Geometry check sheet. Reference: the model listing, model coordinates, mm. A direction names the side the tool comes from. Coordinates: 2 decimals unless noted, no trailing zeros. Order: outer loops, then holes, each group sorted by start corner. A loop starts at its lowest first (then second) coordinate and runs counter-clockwise, first axis right, second up.
```python
from build123d import *

# Parameters (mm, degrees)
SKETCH2_R           = 8
SKETCH2_R_2         = 1.6
SKETCH2_R_3         = 1.5
BOSS_EXTRUDE1_DEPTH = 3


with BuildPart() as part:
    # Sketch2 → Boss-Extrude1 (new body)
    with BuildSketch(Plane.XY):
        with BuildLine():
            Line((118.698481804, 213.752755906), (168.691338583, 213.752755906))
            Line((168.691338583, 213.752755906), (178.691338583, 219.752755906))
            Line((178.691338583, 219.752755906), (258.691338583, 219.752755906))
            Line((258.691338583, 219.752755906), (268.691338583, 213.752755906))
            Line((268.691338583, 213.752755906), (338.214919991, 213.752755906))
            ThreePointArc((338.214919991, 213.752755906), (368.691338583, 289.752755906), (338.214919991, 365.752755906))
            Line((338.214919991, 365.752755906), (268.691338583, 365.752755906))
            Line((268.691338583, 365.752755906), (258.691338583, 359.752755906))
            Line((258.691338583, 359.752755906), (178.691338583, 359.752755906))
            Line((178.691338583, 359.752755906), (168.691338583, 365.752755906))
            Line((168.691338583, 365.752755906), (118.698481804, 365.752755906))
            ThreePointArc((118.698481804, 365.752755906), (111.678103304, 362.874152237), (108.699502265, 355.895613048))
            ThreePointArc((108.699502265, 355.895613048), (109.530508537, 343.195810526), (112.36497097, 330.788499042))
            ThreePointArc((112.36497097, 330.788499042), (123.691338583, 289.752755906), (112.36497097, 248.717012769))
            ThreePointArc((112.36497097, 248.717012769), (109.530508537, 236.309701285), (108.699502265, 223.609898763))
            ThreePointArc((108.699502265, 223.609898763), (111.678103304, 216.631359574), (118.698481804, 213.752755906))
        make_face()
        with Locations((198.291338583, 289.752755906)):
            Circle(SKETCH2_R, mode=Mode.SUBTRACT)
        with Locations((264.091338583, 289.752755906)):
            Circle(SKETCH2_R, mode=Mode.SUBTRACT)
        with Locations((264.091338583, 338.052755906)):
            Circle(SKETCH2_R_2, mode=Mode.SUBTRACT)
        with Locations((260.591338583, 318.752755906)):
            Circle(SKETCH2_R_2, mode=Mode.SUBTRACT)
        with Locations((245.391338583, 311.552755906)):
            Circle(SKETCH2_R_2, mode=Mode.SUBTRACT)
        with Locations((238.791338583, 344.752755906)):
            Circle(SKETCH2_R_2, mode=Mode.SUBTRACT)
        with Locations((239.591338583, 318.752755906)):
            Circle(SKETCH2_R_2, mode=Mode.SUBTRACT)
        with Locations((234.591338583, 312.752755906)):
            Circle(SKETCH2_R_2, mode=Mode.SUBTRACT)
        with Locations((227.791338583, 312.752755906)):
            Circle(SKETCH2_R_2, mode=Mode.SUBTRACT)
        with Locations((216.991338583, 311.552755906)):
            Circle(SKETCH2_R_2, mode=Mode.SUBTRACT)
        with Locations((222.791338583, 318.752755906)):
            Circle(SKETCH2_R_2, mode=Mode.SUBTRACT)
        with Locations((223.591338583, 344.752755906)):
            Circle(SKETCH2_R_2, mode=Mode.SUBTRACT)
        with Locations((201.791338583, 318.752755906)):
            Circle(SKETCH2_R_2, mode=Mode.SUBTRACT)
        with Locations((194.791338583, 318.752755906)):
            Circle(SKETCH2_R_2, mode=Mode.SUBTRACT)
        with Locations((199.100829472, 338.052755906)):
            Circle(SKETCH2_R_2, mode=Mode.SUBTRACT)
        with Locations((191.091338583, 320.252755906)):
            Circle(SKETCH2_R_2, mode=Mode.SUBTRACT)
        with Locations((191.091338583, 314.852755906)):
            Circle(SKETCH2_R_2, mode=Mode.SUBTRACT)
        with Locations((179.591338583, 311.552755906)):
            Circle(SKETCH2_R_2, mode=Mode.SUBTRACT)
        with Locations((173.791338583, 318.752755906)):
            Circle(SKETCH2_R_2, mode=Mode.SUBTRACT)
        with Locations((168.791338583, 312.752755906)):
            Circle(SKETCH2_R_2, mode=Mode.SUBTRACT)
        with Locations((163.691338583, 314.752755906)):
            Circle(SKETCH2_R_3, mode=Mode.SUBTRACT)
        with Locations((163.691338583, 326.752755906)):
            Circle(SKETCH2_R_3, mode=Mode.SUBTRACT)
        with Locations((163.691338583, 338.752755906)):
            Circle(SKETCH2_R_3, mode=Mode.SUBTRACT)
        with Locations((172.991338583, 344.752755906)):
            Circle(SKETCH2_R_2, mode=Mode.SUBTRACT)
        with Locations((163.691338583, 350.752755906)):
            Circle(SKETCH2_R_3, mode=Mode.SUBTRACT)
        with Locations((133.691338583, 350.752755906)):
            Circle(SKETCH2_R_3, mode=Mode.SUBTRACT)
        with Locations((120.691338583, 358.752755906)):
            Circle(SKETCH2_R_3, mode=Mode.SUBTRACT)
        with Locations((117.691338583, 341.752755906)):
            Circle(SKETCH2_R_3, mode=Mode.SUBTRACT)
        with Locations((133.691338583, 338.752755906)):
            Circle(SKETCH2_R_3, mode=Mode.SUBTRACT)
        with Locations((133.691338583, 326.752755906)):
            Circle(SKETCH2_R_3, mode=Mode.SUBTRACT)
        with Locations((133.691338583, 314.752755906)):
            Circle(SKETCH2_R_3, mode=Mode.SUBTRACT)
        with Locations((198.291338583, 241.452755906)):
            Circle(SKETCH2_R_2, mode=Mode.SUBTRACT)
        with Locations((201.791338583, 260.752755906)):
            Circle(SKETCH2_R_2, mode=Mode.SUBTRACT)
        with Locations((216.991338583, 267.952755906)):
            Circle(SKETCH2_R_2, mode=Mode.SUBTRACT)
        with Locations((227.791338583, 266.752755906)):
            Circle(SKETCH2_R_2, mode=Mode.SUBTRACT)
        with Locations((222.791338583, 260.752755906)):
            Circle(SKETCH2_R_2, mode=Mode.SUBTRACT)
        with Locations((223.591338583, 234.752755906)):
            Circle(SKETCH2_R_2, mode=Mode.SUBTRACT)
        with Locations((238.791338583, 234.752755906)):
            Circle(SKETCH2_R_2, mode=Mode.SUBTRACT)
        with Locations((234.591338583, 266.752755906)):
            Circle(SKETCH2_R_2, mode=Mode.SUBTRACT)
        with Locations((245.391338583, 267.952755906)):
            Circle(SKETCH2_R_2, mode=Mode.SUBTRACT)
        with Locations((239.591338583, 260.752755906)):
            Circle(SKETCH2_R_2, mode=Mode.SUBTRACT)
        with Locations((264.091338583, 241.452755906)):
            Circle(SKETCH2_R_2, mode=Mode.SUBTRACT)
        with Locations((260.591338583, 260.752755906)):
            Circle(SKETCH2_R_2, mode=Mode.SUBTRACT)
        with Locations((267.591338583, 260.752755906)):
            Circle(SKETCH2_R_2, mode=Mode.SUBTRACT)
        with Locations((271.291338583, 264.652755906)):
            Circle(SKETCH2_R_2, mode=Mode.SUBTRACT)
        with Locations((271.291338583, 259.252755906)):
            Circle(SKETCH2_R_2, mode=Mode.SUBTRACT)
        with Locations((289.391338583, 234.752755906)):
            Circle(SKETCH2_R_2, mode=Mode.SUBTRACT)
        with Locations((298.691338583, 228.752755906)):
            Circle(SKETCH2_R_3, mode=Mode.SUBTRACT)
        with Locations((298.691338583, 240.752755906)):
            Circle(SKETCH2_R_3, mode=Mode.SUBTRACT)
        with Locations((288.591338583, 260.752755906)):
            Circle(SKETCH2_R_2, mode=Mode.SUBTRACT)
        with Locations((282.791338583, 267.952755906)):
            Circle(SKETCH2_R_2, mode=Mode.SUBTRACT)
        with Locations((293.591338583, 266.752755906)):
            Circle(SKETCH2_R_2, mode=Mode.SUBTRACT)
        with Locations((298.691338583, 264.752755906)):
            Circle(SKETCH2_R_3, mode=Mode.SUBTRACT)
        with Locations((298.691338583, 252.752755906)):
            Circle(SKETCH2_R_3, mode=Mode.SUBTRACT)
        with Locations((328.691338583, 228.752755906)):
            Circle(SKETCH2_R_3, mode=Mode.SUBTRACT)
        with Locations((328.691338583, 240.752755906)):
            Circle(SKETCH2_R_3, mode=Mode.SUBTRACT)
        with Locations((328.691338583, 252.752755906)):
            Circle(SKETCH2_R_3, mode=Mode.SUBTRACT)
        with Locations((328.691338583, 264.752755906)):
            Circle(SKETCH2_R_3, mode=Mode.SUBTRACT)
        with Locations((350.691338583, 244.752755906)):
            Circle(SKETCH2_R_3, mode=Mode.SUBTRACT)
        with Locations((350.691338583, 334.752755906)):
            Circle(SKETCH2_R_3, mode=Mode.SUBTRACT)
        with Locations((328.691338583, 350.752755906)):
            Circle(SKETCH2_R_3, mode=Mode.SUBTRACT)
        with Locations((328.691338583, 338.752755906)):
            Circle(SKETCH2_R_3, mode=Mode.SUBTRACT)
        with Locations((328.691338583, 326.752755906)):
            Circle(SKETCH2_R_3, mode=Mode.SUBTRACT)
        with Locations((328.691338583, 314.752755906)):
            Circle(SKETCH2_R_3, mode=Mode.SUBTRACT)
        with Locations((282.791338583, 311.552755906)):
            Circle(SKETCH2_R_2, mode=Mode.SUBTRACT)
        with Locations((288.591338583, 318.752755906)):
            Circle(SKETCH2_R_2, mode=Mode.SUBTRACT)
        with Locations((293.591338583, 312.752755906)):
            Circle(SKETCH2_R_2, mode=Mode.SUBTRACT)
        with Locations((298.691338583, 314.752755906)):
            Circle(SKETCH2_R_3, mode=Mode.SUBTRACT)
        with Locations((298.691338583, 326.752755906)):
            Circle(SKETCH2_R_3, mode=Mode.SUBTRACT)
        with Locations((298.691338583, 338.752755906)):
            Circle(SKETCH2_R_3, mode=Mode.SUBTRACT)
        with Locations((298.691338583, 350.752755906)):
            Circle(SKETCH2_R_3, mode=Mode.SUBTRACT)
        with Locations((289.391338583, 344.752755906)):
            Circle(SKETCH2_R_2, mode=Mode.SUBTRACT)
        with Locations((271.291338583, 320.252755906)):
            Circle(SKETCH2_R_2, mode=Mode.SUBTRACT)
        with Locations((271.291338583, 314.852755906)):
            Circle(SKETCH2_R_2, mode=Mode.SUBTRACT)
        with Locations((267.591338583, 318.752755906)):
            Circle(SKETCH2_R_2, mode=Mode.SUBTRACT)
        with Locations((120.691338583, 220.752755906)):
            Circle(SKETCH2_R_3, mode=Mode.SUBTRACT)
        with Locations((117.691338583, 237.752755906)):
            Circle(SKETCH2_R_3, mode=Mode.SUBTRACT)
        with Locations((133.691338583, 264.752755906)):
            Circle(SKETCH2_R_3, mode=Mode.SUBTRACT)
        with Locations((133.691338583, 252.752755906)):
            Circle(SKETCH2_R_3, mode=Mode.SUBTRACT)
        with Locations((133.691338583, 240.752755906)):
            Circle(SKETCH2_R_3, mode=Mode.SUBTRACT)
        with Locations((133.691338583, 228.752755906)):
            Circle(SKETCH2_R_3, mode=Mode.SUBTRACT)
        with Locations((163.691338583, 228.752755906)):
            Circle(SKETCH2_R_3, mode=Mode.SUBTRACT)
        with Locations((163.691338583, 240.752755906)):
            Circle(SKETCH2_R_3, mode=Mode.SUBTRACT)
        with Locations((172.991338583, 234.752755906)):
            Circle(SKETCH2_R_2, mode=Mode.SUBTRACT)
        with Locations((163.691338583, 252.752755906)):
            Circle(SKETCH2_R_3, mode=Mode.SUBTRACT)
        with Locations((163.691338583, 264.752755906)):
            Circle(SKETCH2_R_3, mode=Mode.SUBTRACT)
        with Locations((168.791338583, 266.752755906)):
            Circle(SKETCH2_R_2, mode=Mode.SUBTRACT)
        with Locations((173.791338583, 260.752755906)):
            Circle(SKETCH2_R_2, mode=Mode.SUBTRACT)
        with Locations((179.591338583, 267.952755906)):
            Circle(SKETCH2_R_2, mode=Mode.SUBTRACT)
        with Locations((191.091338583, 264.652755906)):
            Circle(SKETCH2_R_2, mode=Mode.SUBTRACT)
        with Locations((194.791338583, 260.752755906)):
            Circle(SKETCH2_R_2, mode=Mode.SUBTRACT)
        with Locations((191.091338583, 259.252755906)):
            Circle(SKETCH2_R_2, mode=Mode.SUBTRACT)
        with BuildLine():
            Line((142.691338583, 297.752755906), (142.691338583, 281.752755906))
            ThreePointArc((142.691338583, 281.752755906), (148.691338583, 275.752755906), (154.691338583, 281.752755906))
            Line((154.691338583, 281.752755906), (154.691338583, 297.752755906))
            ThreePointArc((154.691338583, 297.752755906), (148.691338583, 303.752755906), (142.691338583, 297.752755906))
        make_face(mode=Mode.SUBTRACT)
        with BuildLine():
            Line((307.691338583, 297.752755906), (307.691338583, 281.752755906))
            ThreePointArc((307.691338583, 281.752755906), (313.691338583, 275.752755906), (319.691338583, 281.752755906))
            Line((319.691338583, 281.752755906), (319.691338583, 297.752755906))
            ThreePointArc((319.691338583, 297.752755906), (313.691338583, 303.752755906), (307.691338583, 297.752755906))
        make_face(mode=Mode.SUBTRACT)
        with BuildLine():
            Line((349.191338583, 304.752755906), (349.191338583, 274.752755906))
            ThreePointArc((349.191338583, 274.752755906), (350.691338583, 273.252755906), (352.191338583, 274.752755906))
            Line((352.191338583, 274.752755906), (352.191338583, 304.752755906))
            ThreePointArc((352.191338583, 304.752755906), (350.691338583, 306.252755906), (349.191338583, 304.752755906))
        make_face(mode=Mode.SUBTRACT)
    extrude(amount=BOSS_EXTRUDE1_DEPTH)


solid = part.part
```
Item 1: Sectioned sample at C-C (z = 1.4). Give the number of separate pieces and of enclosed holes in the cut face, and give its area (3 significant figures).
Item 2: Thickness scan on line 1 along X through (y, z) = (254, 2.15); line 2 along X through (y, z) = (283, 2.8); line 3 along Y through (x, z) = (229, 2.7). Record the ranges inside material, lowest first.
Item 3: Tool access check on faces 4 (the face through (148.559, 275.754, 1.479)), 5 (the face through (263.621, 216.795, 1.479)), 6 (the face through (173.76, 362.71, 1.48)), 7 (the face through (123.69, 290.36, 1.48)). Record the directions out of +Z, -Z, +X, -X, +Y, -Y that give a thin tool (end or side, any length) a straight path to the whole face; none if there is none.
Item 4: Depth check by flat-ended pin: P1, Ø2.5, axis at x = 163.69, y = 338.75, coming from the -Z side; P2, Ø0.9, axis at y = 288.5, z = 1, coming from the -X side. Enter the tip coordinate at first touch or a pass-through.
Item 5: Release check for a two-part mould opening along Y. For faces 1 (the face through (173.6, 216.7, 1.5)), 2 (the face through (313.82, 303.75, 1.48)), 3 (the face through (263.761, 362.795, 1.479)) record: pulls with the +Y half, pulls with the -Y half, needs draft (parallel to the pull), parting line crosses it, or undercut.
Item 6: Sectioned sample at B-B (x = 250.5). Record the cut outline in (y, z), and give its area (3 significant figures).
Item 7: Sectioned sample at A-A (x = 316). Record the cut outline in (y, z).
Geometry check:
1. separate pieces: 1
1. enclosed holes: 95
1. area: 34,200 mm2
2. line 1: x = 115.26 to 132.86, 134.52 to 162.86, 164.52 to 297.86, 299.52 to 327.86, 329.52 to 362.72
2. line 2: x = 123.41 to 142.69, 154.69 to 194, 202.58 to 259.8, 268.38 to 307.69, 319.69 to 349.19, 352.19 to 368.48
2. line 3: y = 219.75 to 265.7, 267.8 to 311.7, 313.8 to 359.75
3. face 4: +Z, -Z
3. face 5: +Z, -Z, -Y
3. face 6: +Z, -Z, +Y
3. face 7: +Z, -Z, -X
4. P1: passes through
4. P2: stops at x = 123.67
5. face 1: pulls with the -Y half
5. face 2: undercut
5. face 3: pulls with the +Y half
6. outline: (219.75, 0) - (359.75, 0) - (359.75, 3) - (219.75, 3) - close
6. area: 420 mm2
7. outline: (213.75, 0) - (276.21, 0) - (276.21, 3) - (213.75, 3) - close; (303.29, 0) - (365.75, 0) - (365.75, 3) - (303.29, 3) - close
